The model under review builds one solid part; all positions refer to its coordinate system, in mm. A direction names the side the tool comes from. Coordinates: 2 decimals unless noted, no trailing zeros. Write each loop counter-clockwise with the first axis right and the second up, starting at its lowest first coordinate (ties: lowest second). Pieces come first, ordered by that corner, then holes.
```python
from build123d import *

# Parameters (mm, degrees)
F0_W      = 139.4520141184
F0_H      = 104.3851450086
F1_DEPTH  = 10
F2_W      = 139.4520141184
F2_H      = 34.2989321798
F3_DEPTH  = 50
F4_DEPTH  = 27
F5_DEPTH  = 10
F6_DEPTH  = 25
F7_W      = 53.5153914243
F7_H      = 18.0249847472
F8_DEPTH  = 81
F9_W      = 33.8615532964
F9_H      = 16.5060851723
F10_DEPTH = 258


with BuildPart() as f1:
    # F0 (on Top) → F1 (new body)
    with BuildSketch(Plane.XY):
        with Locations((-1.7260108143, -2.0494647324)):
            Rectangle(F0_W, F0_H)
    extrude(amount=F1_DEPTH)

    # F2 (on face) → F3 (join)
    with BuildSketch(Plane.XY.offset(10)):
        with Locations((-1.7260108143, 32.993641682)):
            Rectangle(F2_W, F2_H)
    extrude(amount=F3_DEPTH)

    # F4 (add): a face of the model
    f4_faces = [f1.faces().sort_by_distance(p)[0] for p in [
        (-1.7260108143, -19.1989308223, 10),
    ]]
    extrude(f4_faces, amount=F4_DEPTH)

    # F5 (add): a face of the model
    f5_faces = [f1.faces().sort_by_distance(p)[0] for p in [
        (-1.7260108143, 32.993641682, 60),
    ]]
    extrude(f5_faces, amount=F5_DEPTH)

    # F6 (cut): a face of the model
    f6_faces = [f1.faces().sort_by_distance(p)[0] for p in [
        (-1.7260108143, -54.2420372367, 18.5),
    ]]
    extrude(f6_faces, amount=-F6_DEPTH, mode=Mode.SUBTRACT)

    # F7 (on face) → F8 (cut)
    with BuildSketch(Plane.XZ.offset(29.2420372367)):
        with Locations((0.5511036143, 9.0124923736)):
            Rectangle(F7_W, F7_H)
    extrude(amount=-F8_DEPTH, mode=Mode.SUBTRACT)

    # F9 (on face) → F10 (cut)
    with BuildSketch(Plane(origin=(-71.4520178735, 0, 0), x_dir=(0, -1, 0), z_dir=(-1, 0, 0))):
        with Locations((-7.9709040001, 8.2530425861)):
            Rectangle(F9_W, F9_H)
    extrude(amount=-F10_DEPTH, mode=Mode.SUBTRACT)


solid = f1.part
```
Item 1: Take a section at C-C, the plane z = 42.5. Write out the cut boundary in (x, y).
Solved:
outline: (-71.45, 15.84) - (68, 15.84) - (68, 50.14) - (-71.45, 50.14) - close
Item 2: To check wall thickness, follow line 1 along X through (y, z) = (38.5, 9); line 2 along Y through (x, z) = (-37.5, 7); line 3 along Z through (x, y) = (32.5, 23.5). State the ranges of each line that lie inside material, in increasing order.
Solved:
line 1: x = -71.45 to -26.21, 27.31 to 68
line 2: y = -29.24 to -8.96, 24.9 to 50.14
line 3: z = 16.51 to 70
Item 3: Mouldability with a two-part tool opening along X and no side actions: class faces 4 (the face through (27.309, 10, 17)), 5 (the face through (-71.452, 19, 35)), 6 (the face through (-26.207, 10, 17)), 7 (the face through (-3, -6, 37)) as pulls with the +X half, pulls with the -X half, needs draft (parallel to the pull), parting line crosses it, or undercut.
Solved:
face 4: undercut
face 5: pulls with the -X half
face 6: undercut
face 7: needs draft
Item 4: Take a section at D-D, the plane y = 23. Write out the cut boundary in (x, z), plus the area to 3 significant figures.
Solved:
outline: (-71.45, 16.51) - (-26.21, 16.51) - (-26.21, 18.02) - (27.31, 18.02) - (27.31, 16.51) - (68, 16.51) - (68, 70) - (-71.45, 70) - close
area: 7,380 mm2
Item 5: For pin 1 (10 mm diameter, centred on x = 44, y = 12, fed in from -Z); pin 2 (8 mm diameter, centred on x = -32, z = 55, fed in from -Y); pin 3 (5 mm diameter, centred on x = 25, y = -12.5, fed in from +Z), all flat-tipped, find the tip position at first contact; note any pin that passes through.
Solved:
pin 1: stops at z = 16.51
pin 2: stops at y = 15.84
pin 3: stops at z = 37
Item 6: Take a section at A-A, the plane y = 6.5. Write out the cut boundary in (x, z), plus the area to 3 significant figures.
Solved:
outline: (-71.45, 16.51) - (-26.21, 16.51) - (-26.21, 18.02) - (27.31, 18.02) - (27.31, 16.51) - (68, 16.51) - (68, 37) - (-71.45, 37) - close
area: 2,780 mm2
Item 7: Machinability: for faces 1 (the face through (-3, 15.844, 53)), 2 (the face through (47, -8.96, 8)), 3 (the face through (-3, 50.143, 35)), which of the approach directions +Z, -Z, +X, -X, +Y, -Y give a long, thin tool a straight path to every point of the face, cutting with its end or side? Answer none if there is none.
Solved:
face 1: +Z, +X, -X, -Y
face 2: -Z, +X, -X
face 3: +Z, -Z, +X, -X, +Y
Item 8: Take a section at B-B, the plane x = -20. Write out the cut boundary in (y, z), plus the area to 3 significant figures.
Solved:
outline: (-29.24, 18.02) - (50.14, 18.02) - (50.14, 70) - (15.84, 70) - (15.84, 37) - (-29.24, 37) - close
area: 2,640 mm2
